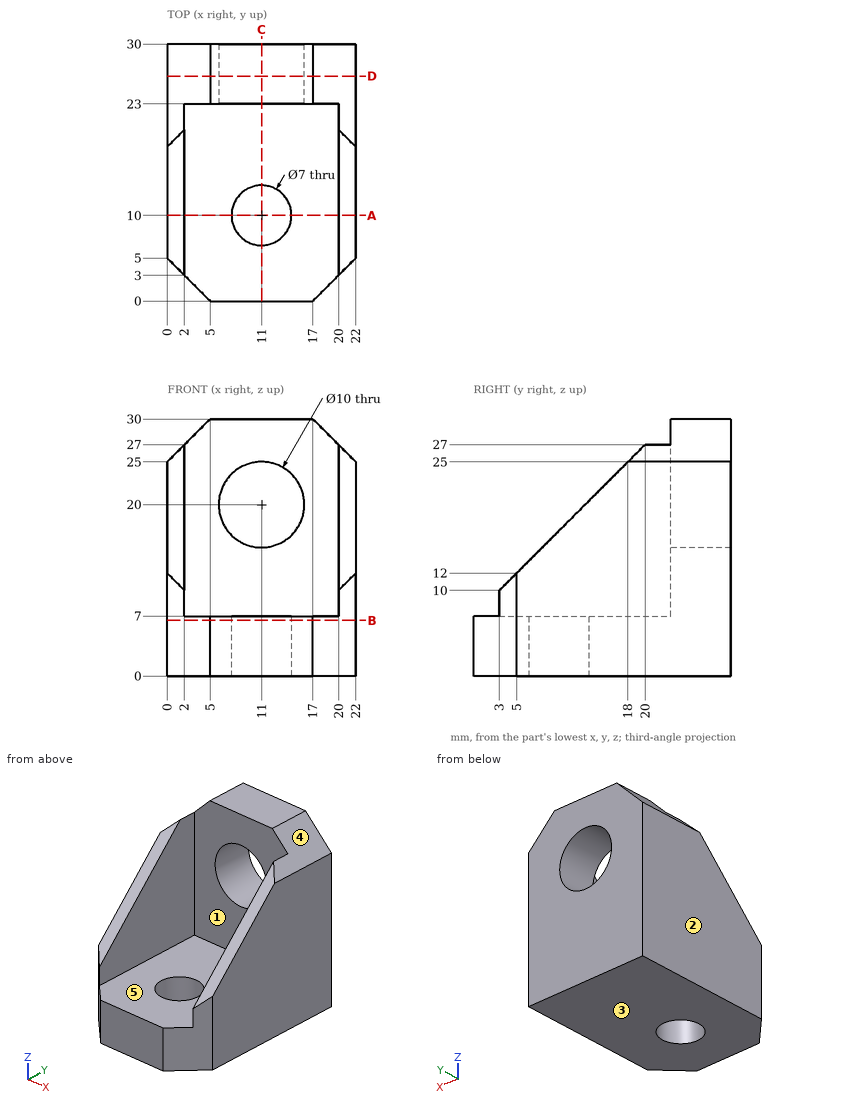
For this review, use the dimensioned drawing (mm, ordinates from the lowest corner) and the shaded views. A direction names the side the tool comes from. Round coordinates to 2 decimals unless told otherwise and drop trailing zeros. Order: outer loops, then holes, each group sorted by start corner. A loop starts at its lowest first (then second) coordinate and runs counter-clockwise, first axis right, second up. Notation, with made-up numbers: M 2.5,76 L 24.5,76 A19 ccw 24.5,85 Z; hole C 10,8 d11. An arc over 180 degrees is marked long. Write each question's results on one line, items separated by ' | '. Start each with the question number.
1. Add section A-A (y = 10). State the section outline as (x, z) points, then the cut area to 3 significant figures.
2. To check wall thickness, follow L1, parallel to Z at x = 11, y = 28.25; L2, parallel to X at y = 14.5, z = 9.5; L3, parallel to Y at x = 18.75, z = 15. State the ranges of each line that lie inside material, in increasing order. Write a range as [from, to].
3. Add section C-C (x = 11). State the section outline as (y, z) points.
4. Add section B-B (z = 6.5). State the section outline as (x, y) points.
5. Tool access review of the marked faces 4 and 5: name each direction out of +Z, -Z, +X, -X, +Y, -Y from which nothing blocks a thin tool from reaching the whole face with its end or side.
6. Clearance check with flat-ended pins moving along their axes: pin 1 Ø4 at (x, y) = (6, 13.5) entering from +Z; pin 2 Ø9 at (x, z) = (13, 19.5) entering from -Y. State where each tip first meets the part, or that it passes through.
7. Draft analysis for pull direction X (two halves, no side actions). For the marked faces 1, 2 and 3, state which applies: pulls with the +X half, pulls with the -X half, needs draft (parallel to the pull), parting line crosses it, or undercut.
8. Add section D-D (y = 26.25). State the section outline as (x, z) points.
Output values:
1) outline: M 0,0 L 7.5,0 L 7.5,7 L 2,7 L 2,17 L 0,17 Z; M 14.5,0 L 22,0 L 22,17 L 20,17 L 20,7 L 14.5,7 Z | area: 145 mm^2
2) L1: [0, 15], [25, 30] | L2: [0, 2], [20, 22] | L3: [23, 30]
3) outline: M 0,0 L 6.5,0 L 6.5,7 L 0,7 Z; M 13.5,0 L 30,0 L 30,15 L 23,15 L 23,7 L 13.5,7 Z; M 23,25 L 30,25 L 30,30 L 23,30 Z
4) outline: M 0,5 L 5,0 L 17,0 L 22,5 L 22,30 L 0,30 Z; hole C 11,10 d7
5) face 4: +Z, +X, +Y, -Y | face 5: +Z, -Y
6) pin 1: z = 7 | pin 2: y = 23
7) face 1: undercut | face 2: pulls with the -X half | face 3: needs draft
8) outline: M 0,0 L 22,0 L 22,25 L 17,30 L 5,30 L 0,25 Z; hole C 11,20 d10
